Input: dimensioned drawing with shaded views. Units: mm. Origin: part minimum x, y, z. A direction names the side the tool comes from. Give positions to 0.01 mm unless a question says otherwise; leave off trailing zeros. Write each loop counter-clockwise with the first axis right and the second up, starting at its lowest first coordinate (ties: lowest second). Pieces come first, ordered by that corner, then holes. Notation, with made-up numbers: (16, 40) - (48, 40) arc R20 cw to (48, 54) - close; hole circle Ø3 at (20.5, -2.5). An arc over 180 degrees is marked (long way). Answer as CSV lines item,"result".
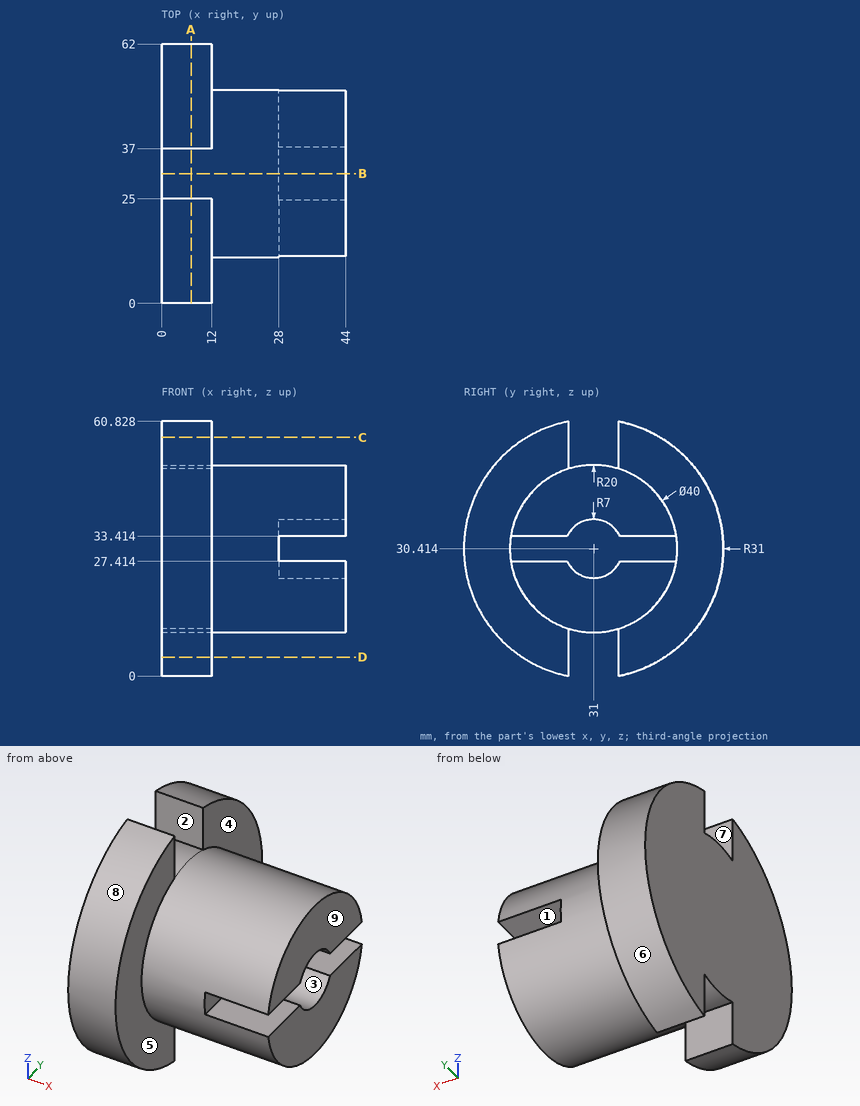
Item 1: Contact query for flat-ended pins moving along their axis: pin 1 (4 mm diameter, centred on x = 40, y = 42.5, fed in from -Z) (1 decimal); pin 2 (4 mm diameter, centred on y = 13.5, z = 23.5, fed in from -X); pin 3 (3 mm diameter, centred on x = 16.5, y = 31.5, fed in from +Z); pin 4 (6 mm diameter, centred on x = 13, y = 9, fed in from -Z). Output: stop coordinate, or through.
The answers:
pin 1,"z = 12.8"
pin 2,"x = 0"
pin 3,"z = 50.41"
pin 4,"z = 6.05"
Item 2: Cut plane C-C on z = 57. Return the cut outline in (x, y).
The answers:
outline,"(0, 15.06) - (12, 15.06) - (12, 25) - (0, 25) - close; (0, 37) - (12, 37) - (12, 46.94) - (0, 46.94) - close"
Item 3: Cut plane D-D on z = 4.5. Return the cut outline in (x, y), plus the area to 3 significant figures.
The answers:
outline,"(0, 13.99) - (12, 13.99) - (12, 25) - (0, 25) - close; (0, 37) - (12, 37) - (12, 48.01) - (0, 48.01) - close"
area,"264 mm²"
Item 4: Reachability of the marked faces 1, 2, 3, 4 and 5 from +Z, -Z, +X, -X, +Y, -Y: full face, straight path, thin tool, end or side. Return the list, or none.
The answers:
face 1,"+X, +Y, -Y"
face 2,"+Z, +X, -X"
face 3,"+X"
face 4,"+X, +Y"
face 5,"+X, -Y"
Item 5: Mould query, pull axis Y, two halves, no side actions, for the marked faces 6, 7, 8 and 9. Classes: +Y half, -Y half, draft (parallel to the pull), parting line (faces both ways), or undercut.
The answers:
face 6,"+Y half"
face 7,"undercut"
face 8,"-Y half"
face 9,"draft"
Item 6: Cut plane B-B on y = 31. Return the cut outline in (x, z), plus the area to 3 significant figures.
The answers:
outline,"(0, 10.41) - (44, 10.41) - (44, 23.41) - (28, 23.41) - (28, 37.41) - (44, 37.41) - (44, 50.41) - (0, 50.41) - close"
area,"1,540 mm²"
Item 7: Ray query, line 1 (X direction, y = 21.5, z = 9); line 2 (X direction, y = 40, z = 28); line 3 (Z direction, x = 31.5, y = 43.5) (1 decimal). Return the intervals inside material, ascending. Write a range as from..to.
The answers:
line 1,"0..12"
line 2,"0..28"
line 3,"14.8..27.4, 33.4..46"
Item 8: Cut plane A-A on x = 7. Return the cut outline in (y, z) (1 decimal), plus the area to 3 significant figures.
The answers:
outline,"(25, 0) - (25, 11.3) arc R20 ccw to (37, 11.3) - (37, 0) arc R31 ccw to (37, 60.8) - (37, 49.5) arc R20 ccw to (25, 49.5) - (25, 60.8) arc R31 ccw to start"
area,"2,750 mm²"
